For this review, take the finished solid that the model builds, in its own axes (mm). Face numbers are marked on the shaded views. Coordinates: 2 decimals unless noted, no trailing zeros. Write each loop counter-clockwise with the first axis right and the second up, starting at its lowest first coordinate (ties: lowest second). Pieces come first, ordered by that corner, then holes. Notation, with made-up numbers: (-25, 26.5) -> (14, 26.5) arc R27 ccw to (14, 62.5) -> close; hole circle Ø2 at (-0.5, 11). An arc over 180 degrees is marked (long way). One line per item, written item: value. Start each with the question number.
1) Add section C-C (z = 7). State the section outline as (x, y) points, and give its area (3 significant figures).
2) Mouldability with a two-part tool opening along Y and no side actions: class the marked faces 1 and 2 as released by +Y, released by -Y, zero draft, split by the parting line, or undercut.
3) Add section A-A (x = 0). State the section outline as (y, z) points.
4) For pin 1 Ø2 at (y, z) = (-1.5, 4) entering from -X; pin 2 Ø8 at (x, y) = (2, -11) entering from +Z; pin 3 Ø2 at (x, y) = (9.5, -10) entering from -Z; pin 4 Ø2 at (x, z) = (5.5, 3.5) entering from +Y, all flat-tipped, find the tip position at first contact; note any pin that passes through.
5) For probe 1 along Y at (x, z) = (0, 4); probe 2 along X at (y, z) = (-8.5, 7.75); probe 3 along X at (y, z) = (1, 8.5), list the stretches that pass through material, from the lowest coordinate up. Write a range as from..to.
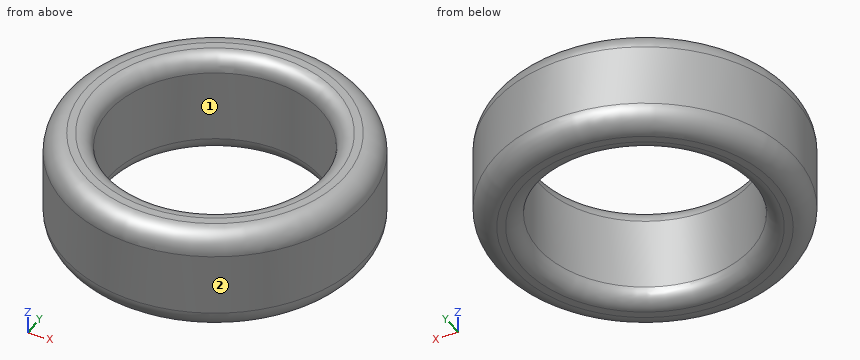
Autodesk Fusion 360 part; units mm, degrees
sketch "Esboço1" plane through (0, 0, 0) normal (0, 0, 1) x (1, 0, 0)
  circle A0 centre (0, 0) radius 10.25
  circle A1 centre (0, 0) radius 14.5
  dimension "d1" = 20.5
  dimension "d2" = 4.25
extrude "Extrusão1" add sketch "Esboço1" along normal blind 10
fillet "Arredondamento1" radius 2 1 edges at (-13.5187, -5.2434, 10)
fillet "Arredondamento2" radius 2 1 edges at (-13.5187, -5.2434, 0)
fillet "Arredondamento3" radius 1.5 1 edges at (-9.5564, 3.7066, 10)
fillet "Arredondamento4" radius 1.5 1 edges at (-9.5564, 3.7066, 0)
Numbers:
1. outline: circle Ø29 at (0, 0); hole circle Ø20.5 at (0, 0)
1. area: 330 mm²
2. face 1: undercut
2. face 2: split by the parting line
3. outline: (-14.5, 2) arc R2 ccw to (-12.5, 0) -> (-11.75, 0) arc R1.5 ccw to (-10.25, 1.5) -> (-10.25, 8.5) arc R1.5 ccw to (-11.75, 10) -> (-12.5, 10) arc R2 ccw to (-14.5, 8) -> close; (10.25, 1.5) arc R1.5 ccw to (11.75, 0) -> (12.5, 0) arc R2 ccw to (14.5, 2) -> (14.5, 8) arc R2 ccw to (12.5, 10) -> (11.75, 10) arc R1.5 ccw to (10.25, 8.5) -> close
4. pin 1: x = -14.49
4. pin 2: z = 10
4. pin 3: z = 0.02
4. pin 4: y = 13.78
5. probe 1: -14.5..-10.25, 10.25..14.5
5. probe 2: -11.75..-5.73, 5.73..11.75
5. probe 3: -14.4..-10.2, 10.2..14.4
